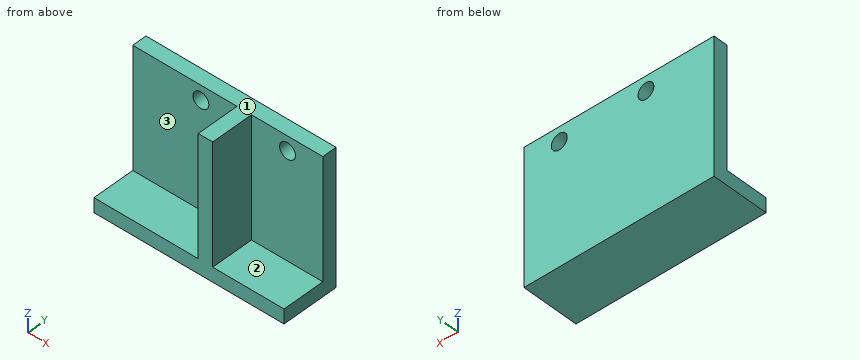
Autodesk Inventor part; units mm, degrees
ref_plane "YZ Plane" through (0, 0, 0) normal (1, 0, 0) x (0, 1, 0)
ref_plane "XZ Plane" through (0, 0, 0) normal (0, 1, 0) x (-1, 0, 0)
ref_plane "XY Plane" through (0, 0, 0) normal (0, 0, 1) x (1, 0, 0)
sketch "Sketch1" plane through (0, 0, 0) normal (0, 0, 1) x (1, 0, 0)
  line L0 (-109, -87.5) -> (109, -87.5)
  line L1 (109, -87.5) -> (109, 87.5)
  line L2 (109, 87.5) -> (-109, 87.5)
  line L3 (-109, 87.5) -> (-109, -87.5)
  line L4 (-109, -87.5) -> (109, 87.5) construction
  line L5 (109, -87.5) -> (-109, 87.5) construction
  point P0 (0, 0)
  dimension "d0" = 218
  dimension "d1" = 175
extrude "Extrusion1" add sketch "Sketch1" along normal blind 28
sketch "Sketch2" plane through (0, 0, 28) normal (0, 0, 1) x (1, 0, 0)
  line L0 (-106, 84.5) -> (-66, 84.5)
  line L1 (-66, 84.5) -> (-66, 44.5)
  line L2 (-66, 44.5) -> (-106, 44.5)
  line L3 (-106, 44.5) -> (-106, 84.5)
  line L4 (-106, 84.5) -> (-66, 44.5) construction
  line L5 (-66, 84.5) -> (-106, 44.5) construction
  line L6 (109, 87.5) -> (-109, 87.5)
  line L7 (-109, 87.5) -> (-109, -87.5)
  line L8 (-63, 84.5) -> (-23, 84.5)
  line L9 (-23, 84.5) -> (-23, 44.5)
  line L10 (-23, 44.5) -> (-63, 44.5)
  line L11 (-63, 44.5) -> (-63, 84.5)
  line L12 (-63, 84.5) -> (-23, 44.5) construction
  line L13 (-23, 84.5) -> (-63, 44.5) construction
  line L14 (-20, 84.5) -> (20, 84.5)
  line L15 (20, 84.5) -> (20, 44.5)
  line L16 (20, 44.5) -> (-20, 44.5)
  line L17 (-20, 44.5) -> (-20, 84.5)
  line L18 (-20, 84.5) -> (20, 44.5) construction
  line L19 (20, 84.5) -> (-20, 44.5) construction
  line L20 (23, 84.5) -> (63, 84.5)
  line L21 (63, 84.5) -> (63, 44.5)
  line L22 (63, 44.5) -> (23, 44.5)
  line L23 (23, 44.5) -> (23, 84.5)
  line L24 (23, 84.5) -> (63, 44.5) construction
  line L25 (63, 84.5) -> (23, 44.5) construction
  line L26 (66, 84.5) -> (106, 84.5)
  line L27 (106, 84.5) -> (106, 44.5)
  line L28 (106, 44.5) -> (66, 44.5)
  line L29 (66, 44.5) -> (66, 84.5)
  line L30 (66, 84.5) -> (106, 44.5) construction
  line L31 (106, 84.5) -> (66, 44.5) construction
  line L32 (-106, 41.5) -> (-66, 41.5)
  line L33 (-66, 41.5) -> (-66, 1.5)
  line L34 (-66, 1.5) -> (-106, 1.5)
  line L35 (-106, 1.5) -> (-106, 41.5)
  line L36 (-106, 41.5) -> (-66, 1.5) construction
  line L37 (-66, 41.5) -> (-106, 1.5) construction
  line L38 (-63, 41.5) -> (-23, 41.5)
  line L39 (-23, 41.5) -> (-23, 1.5)
  line L40 (-23, 1.5) -> (-63, 1.5)
  line L41 (-63, 1.5) -> (-63, 41.5)
  line L42 (-63, 41.5) -> (-23, 1.5) construction
  line L43 (-23, 41.5) -> (-63, 1.5) construction
  line L44 (-20, 41.5) -> (20, 41.5)
  line L45 (20, 41.5) -> (20, 1.5)
  line L46 (20, 1.5) -> (-20, 1.5)
  line L47 (-20, 1.5) -> (-20, 41.5)
  line L48 (-20, 41.5) -> (20, 1.5) construction
  line L49 (20, 41.5) -> (-20, 1.5) construction
  line L50 (23, 41.5) -> (63, 41.5)
  line L51 (63, 41.5) -> (63, 1.5)
  line L52 (63, 1.5) -> (23, 1.5)
  line L53 (23, 1.5) -> (23, 41.5)
  line L54 (23, 41.5) -> (63, 1.5) construction
  line L55 (63, 41.5) -> (23, 1.5) construction
  line L56 (66, 41.5) -> (106, 41.5)
  line L57 (106, 41.5) -> (106, 1.5)
  line L58 (106, 1.5) -> (66, 1.5)
  line L59 (66, 1.5) -> (66, 41.5)
  line L60 (66, 41.5) -> (106, 1.5) construction
  line L61 (106, 41.5) -> (66, 1.5) construction
  line L62 (-106, -1.5) -> (-66, -1.5)
  line L63 (-66, -1.5) -> (-66, -41.5)
  line L64 (-66, -41.5) -> (-106, -41.5)
  line L65 (-106, -41.5) -> (-106, -1.5)
  line L66 (-106, -1.5) -> (-66, -41.5) construction
  line L67 (-66, -1.5) -> (-106, -41.5) construction
  line L68 (-63, -1.5) -> (-23, -1.5)
  line L69 (-23, -1.5) -> (-23, -41.5)
  line L70 (-23, -41.5) -> (-63, -41.5)
  line L71 (-63, -41.5) -> (-63, -1.5)
  line L72 (-63, -1.5) -> (-23, -41.5) construction
  line L73 (-23, -1.5) -> (-63, -41.5) construction
  line L74 (-20, -1.5) -> (20, -1.5)
  line L75 (20, -1.5) -> (20, -41.5)
  line L76 (20, -41.5) -> (-20, -41.5)
  line L77 (-20, -41.5) -> (-20, -1.5)
  line L78 (-20, -1.5) -> (20, -41.5) construction
  line L79 (20, -1.5) -> (-20, -41.5) construction
  line L80 (23, -1.5) -> (63, -1.5)
  line L81 (63, -1.5) -> (63, -41.5)
  line L82 (63, -41.5) -> (23, -41.5)
  line L83 (23, -41.5) -> (23, -1.5)
  line L84 (23, -1.5) -> (63, -41.5) construction
  line L85 (63, -1.5) -> (23, -41.5) construction
  line L86 (66, -1.5) -> (106, -1.5)
  line L87 (106, -1.5) -> (106, -41.5)
  line L88 (106, -41.5) -> (66, -41.5)
  line L89 (66, -41.5) -> (66, -1.5)
  line L90 (66, -1.5) -> (106, -41.5) construction
  line L91 (106, -1.5) -> (66, -41.5) construction
  line L92 (-106, -44.5) -> (-66, -44.5)
  line L93 (-66, -44.5) -> (-66, -84.5)
  line L94 (-66, -84.5) -> (-106, -84.5)
  line L95 (-106, -84.5) -> (-106, -44.5)
  line L96 (-106, -44.5) -> (-66, -84.5) construction
  line L97 (-66, -44.5) -> (-106, -84.5) construction
  line L98 (-63, -44.5) -> (-23, -44.5)
  line L99 (-23, -44.5) -> (-23, -84.5)
  line L100 (-23, -84.5) -> (-63, -84.5)
  line L101 (-63, -84.5) -> (-63, -44.5)
  line L102 (-63, -44.5) -> (-23, -84.5) construction
  line L103 (-23, -44.5) -> (-63, -84.5) construction
  line L104 (-20, -44.5) -> (20, -44.5)
  line L105 (20, -44.5) -> (20, -84.5)
  line L106 (20, -84.5) -> (-20, -84.5)
  line L107 (-20, -84.5) -> (-20, -44.5)
  line L108 (-20, -44.5) -> (20, -84.5) construction
  line L109 (20, -44.5) -> (-20, -84.5) construction
  line L110 (23, -44.5) -> (63, -44.5)
  line L111 (63, -44.5) -> (63, -84.5)
  line L112 (63, -84.5) -> (23, -84.5)
  line L113 (23, -84.5) -> (23, -44.5)
  line L114 (23, -44.5) -> (63, -84.5) construction
  line L115 (63, -44.5) -> (23, -84.5) construction
  line L116 (66, -44.5) -> (106, -44.5)
  line L117 (106, -44.5) -> (106, -84.5)
  line L118 (106, -84.5) -> (66, -84.5)
  line L119 (66, -84.5) -> (66, -44.5)
  line L120 (66, -44.5) -> (106, -84.5) construction
  line L121 (106, -44.5) -> (66, -84.5) construction
  point P0 (0, 0)
  point P1 (-86, 64.5)
  point P2 (-43, 64.5)
  point P3 (0, 64.5)
  point P4 (43, 64.5)
  point P5 (86, 64.5)
  point P6 (-86, 21.5)
  point P7 (-43, 21.5)
  point P8 (0, 21.5)
  point P9 (43, 21.5)
  point P10 (86, 21.5)
  point P11 (-86, -21.5)
  point P12 (-43, -21.5)
  point P13 (0, -21.5)
  point P14 (43, -21.5)
  point P15 (86, -21.5)
  point P16 (-86, -64.5)
  point P17 (-43, -64.5)
  point P18 (0, -64.5)
  point P19 (43, -64.5)
  point P20 (86, -64.5)
  dimension "d4" = 40
  dimension "d5" = 3
  dimension "d6" = 3
  dimension "d7" = 40
  dimension "d10" = 43
  dimension "d13" = 43
extrude "Extrusion2" cut sketch "Sketch2" against normal blind 25
sketch "Sketch3" plane through (-109, 87.5, 0) normal (0, 1, 0) x (1, 0, 0)
  line L0 (46, -28) -> (46, -3) construction
  line L1 (43, -28) -> (43, -3) construction
  line L2 (43, -28) -> (43, -3)
  line L3 (43, -25) -> (46, -25) construction
  line L4 (46, -28) -> (46, -3)
  line L5 (218, -28) -> (0, -28)
  circle A0 centre (53.5, -25) radius 1.65
  circle A1 centre (35.5, -25) radius 1.65
  line L6 (172, -28) -> (172, -3) construction
  line L7 (175, -28) -> (175, -3) construction
  line L8 (172, -28) -> (172, -3)
  line L9 (172, -25) -> (175, -25) construction
  circle A2 centre (182.5, -25) radius 1.65
  circle A3 centre (164.5, -25) radius 1.65
  point P0 (109, 0)
  point P1 (44.5, -25)
  point P2 (173.5, -25)
  dimension "d20" = 3
  dimension "d21" = 3.3
  dimension "d22" = 9
  dimension "d23" = 3.3
  dimension "d24" = 9
  dimension "d25" = 3.3
  dimension "d27" = 9
  dimension "d30" = 3
  dimension "d31" = 3.3
  dimension "d32" = 9
extrude "Extrusion3" cut sketch "Sketch3" against normal blind 10
sketch "Sketch4" plane through (0, 0, 0) normal (0, 0, -1) x (-1, 0, 0)
  line L0 (-109, 87.5) -> (109, 87.5)
  line L1 (48.1771, 87.5) -> (-137.115, 87.5)
  line L2 (-137.115, 87.5) -> (-137.115, -97.6556)
  line L3 (-137.115, -97.6556) -> (48.1771, -97.6556)
  line L4 (48.1771, -97.6556) -> (48.1771, 87.5)
  line L5 (153.7374, -115.3645) -> (-15.4329, -115.3645)
  line L6 (-15.4329, -115.3645) -> (-15.4329, 75.6885)
  line L7 (-15.4329, 75.6885) -> (153.7374, 75.6885)
  line L8 (153.7374, 75.6885) -> (153.7374, -115.3645)
  line L9 (153.7374, 38.7258) -> (87.6444, 38.7258)
  line L10 (87.6444, 38.7258) -> (87.6444, 105.9246)
  line L11 (87.6444, 105.9246) -> (153.7374, 105.9246)
  line L12 (153.7374, 105.9246) -> (153.7374, 38.7258)
  point P0 (0, 0)
  point P1 (87.6444, 75.6885)
  point P2 (48.1771, 75.6885)
  point P3 (-15.4329, -97.6556)
  point P4 (153.7374, 75.6885)
extrude "Extrusion4" cut sketch "Sketch4" against normal through all contours L0 L4 L7 L6 L3 L2 L1 | L10 L11 L12 L7 | L7 L10 L9 L8 L5 L6 L3 L4 | L4 L3 L6 L7 | L7 L8 L9 L10
equation "\"d0\" = box_length"
equation "\"d1\" = box_width"
equation "\"d2\" = hole_height + wall"
equation "\"d4\" = hole"
equation "\"d5\" = wall"
equation "\"d6\" = wall"
equation "\"d7\" = hole"
equation "\"d10\" = hole + wall"
equation "\"d13\" = hole + wall"
equation "\"d16\" = hole_height"
equation "\"d23\" = d21"
equation "\"d25\" = d21"
equation "\"d31\" = d25"
equation "\"hole\" = 40"
equation "\"wall\" = 3"
equation "\"hole_height\" = 25"
properties part number "RatPelletBox_v02_holetest"
Check sheet for the modelled part. Datum: model origin and axes. Units: mm. Face numbers are marked on the shaded views. A direction names the side the tool comes from. Round coordinates to 2 decimals unless told otherwise and drop trailing zeros. Loops run counter-clockwise (first coordinate to the right, second up) from the corner with the lowest first, then second, coordinate; pieces in that order, holes last. Notation, with made-up numbers: (81.5, 25) -> (137.5, 25) arc R22 ccw to (137.5, 41) -> close; hole circle Ø6 at (-33, -38). An arc over 180 degrees is marked (long way). Answer in a Markdown table with one row per item.
Q1. Set-up check for the marked faces 1, 2 and 3: record each of +Z, -Z, +X, -X, +Y, -Y from which the full face is reachable in a straight line by a thin tool's end or side.
Data:
| item | result |
|---|---|
| face 1 | +Z, +X, -X, +Y, -Y |
| face 2 | +Z, +X, -Y |
| face 3 | +Z, -X, -Y |
Q2. Go/stop test with flat-tipped pins: P1, Ø4.5, axis at y = 82, z = 20.5, coming from the +X side; P2, Ø2.5, axis at x = -77.5, y = 82, coming from the +Z side; P3, Ø1.5, axis at y = 81, z = 4.5, coming from the -X side. Record where each tip stops, or that it passes through.
Data:
| item | result |
|---|---|
| P1 | stops at x = -63 |
| P2 | stops at z = 3 |
| P3 | stops at x = -66 |
Q3. Sectioned sample at A-A on x = -73.5. Enter the section's corners in (y, z), then the cut area to 3 significant figures.
Data:
| item | result |
|---|---|
| outline | (75.69, 0) -> (87.5, 0) -> (87.5, 23.35) -> (84.5, 23.35) -> (84.5, 3) -> (75.69, 3) -> close; (84.5, 26.65) -> (87.5, 26.65) -> (87.5, 28) -> (84.5, 28) -> close |
| area | 101 mm^2 |
Q4. Sectioned sample at B-B on z = 25. Enter the section's corners in (x, y).
Data:
| item | result |
|---|---|
| outline | (-87.64, 84.5) -> (-75.15, 84.5) -> (-75.15, 87.5) -> (-87.64, 87.5) -> close; (-71.85, 84.5) -> (-66, 84.5) -> (-66, 75.69) -> (-63, 75.69) -> (-63, 84.5) -> (-57.15, 84.5) -> (-57.15, 87.5) -> (-71.85, 87.5) -> close; (-53.85, 84.5) -> (-48.18, 84.5) -> (-48.18, 87.5) -> (-53.85, 87.5) -> close |
Q5. Thickness scan on L1, parallel to X at y = 85.3, z = 25; L2, parallel to Z at x = -55.5, y = 85.25; L3, parallel to X at y = 85.75, z = 25.75. Record the ranges inside material, lowest first.
Data:
| item | result |
|---|---|
| L1 | x = -87.64 to -75.15, -71.85 to -57.15, -53.85 to -48.18 |
| L2 | z = 0 to 23.35, 26.65 to 28 |
| L3 | x = -87.64 to -74.97, -72.03 to -56.97, -54.03 to -48.18 |
Q6. Sectioned sample at D-D on z = 16.75. Enter the section's corners in (x, y).
Data:
| item | result |
|---|---|
| outline | (-87.64, 84.5) -> (-66, 84.5) -> (-66, 75.69) -> (-63, 75.69) -> (-63, 84.5) -> (-48.18, 84.5) -> (-48.18, 87.5) -> (-87.64, 87.5) -> close |
Q7. Sectioned sample at C-C on y = 82.5. Enter the section's corners in (x, z), then the cut area to 3 significant figures.
Data:
| item | result |
|---|---|
| outline | (-87.64, 0) -> (-48.18, 0) -> (-48.18, 3) -> (-63, 3) -> (-63, 28) -> (-66, 28) -> (-66, 3) -> (-87.64, 3) -> close |
| area | 193 mm^2 |
